```python
from build123d import *

# Parameters (mm, degrees)
SZKIC1_R                    = 2.75
SZKIC1_R_2                  = 2.25
DODANIE_WYCI_GNI_CIE1_DEPTH = 3
ZAOKR_GLENIE1_R             = 3
ZAOKR_GLENIE2_R             = 3


with BuildPart() as part:
    # Szkic1 → Dodanie-wyciągnięcie1 (new body)
    with BuildSketch(Plane.XY):
        Polygon((8.371402008, 50.388834407), (-31.628597992, 50.388834407), (-31.628597992, 10.388834407), (-31.628597992, -9.611165593), (-11.628597992, -9.611165593), (28.371402008, -9.611165593), (28.371402008, 30.388834407), (8.371402008, 30.388834407), align=None)
        with Locations((-21.628597992, 0.388834407)):
            Circle(SZKIC1_R, mode=Mode.SUBTRACT)
        with Locations((-1.628597992, 0.388834407)):
            Circle(SZKIC1_R, mode=Mode.SUBTRACT)
        with Locations((18.371402008, 0.388834407)):
            Circle(SZKIC1_R_2, mode=Mode.SUBTRACT)
        with Locations((-21.628597992, 20.388834407)):
            Circle(SZKIC1_R_2, mode=Mode.SUBTRACT)
        with Locations((-21.628597992, 40.388834407)):
            Circle(SZKIC1_R_2, mode=Mode.SUBTRACT)
        with Locations((-1.628597992, 20.388834407)):
            Circle(SZKIC1_R_2, mode=Mode.SUBTRACT)
        with Locations((18.371402008, 20.388834407)):
            Circle(SZKIC1_R_2, mode=Mode.SUBTRACT)
        with Locations((-1.628597992, 40.388834407)):
            Circle(SZKIC1_R_2, mode=Mode.SUBTRACT)
    extrude(amount=DODANIE_WYCI_GNI_CIE1_DEPTH)

    # Zaokrąglenie1
    zaokr_glenie1_edges = [part.edges().sort_by_distance(p)[0] for p in [
        (-31.628597992, -9.611165593, 1.5),
        (-31.628597992, 50.388834407, 1.5),
        (8.371402008, 50.388834407, 1.5),
        (28.371402008, 30.388834407, 1.5),
        (28.371402008, -9.611165593, 1.5),
    ]]
    fillet(zaokr_glenie1_edges, radius=ZAOKR_GLENIE1_R)

    # Zaokrąglenie2
    zaokr_glenie2_edges = [part.edges().sort_by_distance(p)[0] for p in [
        (8.371402008, 30.388834407, 1.5),
    ]]
    fillet(zaokr_glenie2_edges, radius=ZAOKR_GLENIE2_R)


solid = part.part
```
The listing builds one solid part. Answer for the finished solid, in the listing's coordinates (mm). A direction names the side the tool comes from. Coordinates: 2 decimals unless noted, no trailing zeros. Write each loop counter-clockwise with the first axis right and the second up, starting at its lowest first coordinate (ties: lowest second). Pieces come first, ordered by that corner, then holes.
Q1. Which of the six approach directions +Z, -Z, +X, -X, +Y, -Y give full straight-line access (tool end or side, diameter ignored) to faces 1 (the cylindrical face through (20.52, 1.06, 1.48)), 2 (the flat face through (8.371, 40, 1))?
Returned:
face 1: +Z, -Z
face 2: +Z, -Z, +X, +Y
Q2. Section C-C, the plane y = 35 is taken. Write down the section's boundary in (x, z), then the cut area to 3 significant figures.
Returned:
outline: (-31.63, 0) - (8.37, 0) - (8.37, 3) - (-31.63, 3) - close
area: 120 mm2
Q3. Given P1, Ø0.9, axis at x = 19.5, z = 2, coming from the +Y side, flat-ended and moving along its own axis, determine where the tip first touches the part or whether it passes through.
Returned:
P1: stops at y = 30.39
Q4. Find the intervals of material crossed by line 1 along X through (y, z) = (0.5, 1.25); line 2 along Y through (x, z) = (-21, 1.5); line 3 along X through (y, z) = (1, 0.95), in increasing order.
Returned:
line 1: x = -31.63 to -24.38, -18.88 to -4.38, 1.12 to 16.12, 20.62 to 28.37
line 2: y = -9.61 to -2.29, 3.07 to 18.23, 22.55 to 38.23, 42.55 to 50.39
line 3: x = -31.63 to -24.31, -18.95 to -4.31, 1.05 to 16.21, 20.54 to 28.37
Q5. Section D-D, the plane x = 22.5 is taken. Write down the section's boundary in (y, z).
Returned:
outline: (-9.61, 0) - (30.39, 0) - (30.39, 3) - (-9.61, 3) - close
Q6. Section B-B, the plane z = 0.75 is taken. Give the number of separate pieces and of enclosed holes in the cut face, then the cut area to 3 significant figures.
Returned:
separate pieces: 1
enclosed holes: 8
area: 3,050 mm2
Q7. Section A-A, the plane y = -1 is taken. Write down the section's boundary in (x, z), then the cut area to 3 significant figures.
Returned:
outline: (-31.63, 0) - (-24, 0) - (-24, 3) - (-31.63, 3) - close; (-19.26, 0) - (-4, 0) - (-4, 3) - (-19.26, 3) - close; (0.74, 0) - (16.6, 0) - (16.6, 3) - (0.74, 3) - close; (20.14, 0) - (28.37, 0) - (28.37, 3) - (20.14, 3) - close
area: 141 mm2
